Input: part model. Units: mm. Frame: model coordinates. A direction names the side the tool comes from. Coordinates: 2 decimals unless noted, no trailing zeros. Loops run counter-clockwise (first coordinate to the right, second up) from the corner with the lowest first, then second, coordinate; pieces in that order, holes last.
```python
from build123d import *

# Parameters (mm, degrees)
RESSALTO_EXTRUS_O2_DEPTH = 25
ESBO_O5_R                = 4
CORTE_EXTRUS_O3_DEPTH    = 85
ESBO_O6_R                = 7
CORTE_EXTRUS_O4_DEPTH    = 20
ESBO_O12_W               = 15
ESBO_O12_H               = 110
RESSALTO_EXTRUS_O3_DEPTH = 20
ESBO_O13_W               = 110
ESBO_O13_H               = 110
RESSALTO_EXTRUS_O4_DEPTH = 15
ESBO_O14_R               = 25
ESBO_O14_R_2             = 4
CORTE_EXTRUS_O5_DEPTH    = 15


with BuildPart() as part:
    # Esboço1 → Ressalto-extrusão2 (new body)
    with BuildSketch(Plane.XY):
        with BuildLine():
            Line((6.820228442, 22.38699838), (6.820228442, 18.727313079))
            ThreePointArc((6.820228442, 18.727313079), (19.00741694, -1.705466141), (1.689928033, -18.018976127))
            Line((1.689928033, -18.018976127), (1.689928033, -54.024230705))
            Line((1.689928033, -54.024230705), (55.189928033, -54.024230705))
            Line((55.189928033, -54.024230705), (55.189928033, 55.975769295))
            Line((55.189928033, 55.975769295), (1.689928033, 55.975769295))
            Line((1.689928033, 55.975769295), (-1.310071967, 55.975769295))
            Line((-1.310071967, 55.975769295), (-54.810071967, 55.975769295))
            Line((-54.810071967, 55.975769295), (-54.810071967, -54.024230705))
            Line((-54.810071967, -54.024230705), (-1.310071967, -54.024230705))
            Line((-1.310071967, -54.024230705), (-1.310071967, -18.018976127))
            ThreePointArc((-1.310071967, -18.018976127), (-18.627560875, -1.705466141), (-6.440372377, 18.727313079))
            Line((-6.440372377, 18.727313079), (-6.440372377, 22.38699838))
            Line((-6.440372377, 22.38699838), (6.180238055, 22.38699838))
            Line((6.180238055, 22.38699838), (6.820228442, 22.38699838))
        make_face()
    extrude(amount=RESSALTO_EXTRUS_O2_DEPTH)

    # Esboço5 → Corte-extrusão3 (cut)
    with BuildSketch(Plane.ZY.offset(54.810071967)):
        with Locations((12.5, -41.024230705)):
            Circle(ESBO_O5_R)
    extrude(amount=-CORTE_EXTRUS_O3_DEPTH, mode=Mode.SUBTRACT)

    # Esboço6 → Corte-extrusão4 (cut)
    with BuildSketch(Plane.ZY.offset(54.810071967)):
        with Locations((12.5, -41.024230705)):
            Circle(ESBO_O6_R)
    extrude(amount=-CORTE_EXTRUS_O4_DEPTH, mode=Mode.SUBTRACT)

    # Esboço12 → Ressalto-extrusão3 (add)
    with BuildSketch(Plane.XY.offset(25)):
        with Locations((47.689928033, 0.975769295)):
            Rectangle(ESBO_O12_W, ESBO_O12_H)
    extrude(amount=RESSALTO_EXTRUS_O3_DEPTH)

    # Esboço13 → Ressalto-extrusão4 (add)
    with BuildSketch(Plane.XY.offset(45)):
        with Locations((0.189928033, 0.975769295)):
            Rectangle(ESBO_O13_W, ESBO_O13_H)
    extrude(amount=RESSALTO_EXTRUS_O4_DEPTH)

    # Esboço14 → Corte-extrusão5 (cut)
    with BuildSketch(Plane.XY.offset(60)):
        Circle(ESBO_O14_R)
        with Locations((0, 40)):
            Circle(ESBO_O14_R_2)
        with Locations((-40, 0)):
            Circle(ESBO_O14_R_2)
        with Locations((0, -40)):
            Circle(ESBO_O14_R_2)
        with Locations((-28.284271247, 28.284271247)):
            Circle(ESBO_O14_R_2)
        with Locations((28.284271247, 28.284271247)):
            Circle(ESBO_O14_R_2)
        with Locations((28.284271247, -28.284271247)):
            Circle(ESBO_O14_R_2)
        with Locations((-28.284271247, -28.284271247)):
            Circle(ESBO_O14_R_2)
    extrude(amount=-CORTE_EXTRUS_O5_DEPTH, mode=Mode.SUBTRACT)


solid = part.part
```
Item 1: Contact query for flat-ended pins moving along their axis: P1, Ø10.5, axis at y = -41.02, z = 12.5, coming from the -X side; P2, Ø3, axis at x = -23, z = 27.5, coming from the +Y side. Output: stop coordinate, or through.
Result:
P1: stops at x = -34.81
P2: passes through
Item 2: Section query A-A (z = 12.5). Output: boundary loops of the cut face in (x, y).
Result:
outline: (-54.81, -54.02) - (-1.31, -54.02) - (-1.31, -45.02) - (-34.81, -45.02) - (-34.81, -48.02) - (-54.81, -48.02) - close; (-54.81, -34.02) - (-34.81, -34.02) - (-34.81, -37.02) - (-1.31, -37.02) - (-1.31, -18.02) arc R19 cw to (-6.44, 18.73) - (-6.44, 22.39) - (6.82, 22.39) - (6.82, 18.73) arc R19 cw to (1.69, -18.02) - (1.69, -37.02) - (30.19, -37.02) - (30.19, -45.02) - (1.69, -45.02) - (1.69, -54.02) - (55.19, -54.02) - (55.19, 55.98) - (-54.81, 55.98) - close
Item 3: Mould query, pull axis X, two halves, no side actions, for faces 6 (the face through (-31.23, 30.99, 52.6)), 7 (the face through (-44.95, -35.12, 16.26)), 8 (the face through (-54.81, 2, 12)), 9 (the face through (-32.28, -28.11, 52.6)). Classes: +X half, -X half, draft (parallel to the pull), parting line (faces both ways), or undercut.
Result:
face 6: undercut
face 7: draft
face 8: -X half
face 9: undercut
Item 4: Section query C-C (x = 16.5). Output: boundary loops of the cut face in (y, z).
Result:
outline: (-54.02, 0) - (-8.82, 0) - (-8.82, 25) - (-54.02, 25) - close; (-54.02, 45) - (-18.78, 45) - (-18.78, 60) - (-54.02, 60) - close; (10.67, 0) - (55.98, 0) - (55.98, 25) - (10.67, 25) - close; (18.78, 45) - (55.98, 45) - (55.98, 60) - (18.78, 60) - close; hole circle Ø8 at (-41.02, 12.5)
Item 5: Line query: L1, parallel to Z at x = -43.5, y = 25; L2, parallel to Y at x = 0, z = 50.75; L3, parallel to X at y = -39.5, z = 50.5. Output: solid intervals per line, ascending.
Result:
L1: z = 0 to 25, 45 to 60
L2: y = -54.02 to -44, -36 to -25, 25 to 36, 44 to 55.98
L3: x = -54.81 to -3.97, 3.97 to 55.19
Item 6: Section query D-D (z = 47). Count the separate pieces of the cut face and the enclosed holes in it, then the cut area to 3 significant figures.
Result:
separate pieces: 1
enclosed holes: 8
area: 9,780 mm2
Item 7: Reachability of faces 1 (the face through (-1.31, -36, 12)), 2 (the face through (-34.81, -44, 16)), 3 (the face through (6.82, 21, 12)), 4 (the face through (30.43, 31.66, 52.6)), 5 (the face through (40.19, 0, 35)) from +Z, -Z, +X, -X, +Y, -Y: full face, straight path, thin tool, end or side. Return the list, or none.
Result:
face 1: -Z, -Y
face 2: -X
face 3: +Z, -Z
face 4: +Z
face 5: -X, +Y, -Y
Item 8: Section query B-B (y = 30). Output: boundary loops of the cut face in (x, z).
Result:
outline: (-54.81, 0) - (55.19, 0) - (55.19, 60) - (31.9, 60) - (31.9, 45) - (40.19, 45) - (40.19, 25) - (-54.81, 25) - close; (-54.81, 45) - (-31.9, 45) - (-31.9, 60) - (-54.81, 60) - close; (-24.67, 45) - (24.67, 45) - (24.67, 60) - (-24.67, 60) - close
